from build123d import *

# Parameters (mm, degrees)
SKETCH1_R                          = 61.595
BOSS_EXTRUDE1_DEPTH                = 1.5875
F_1_4_0_25_DIAMETER_HOLE1_D        = 6.35
F_5_16_0_3125_DIAMETER_HOLE1_D     = 7.9375
F_5_16_0_3125_DIAMETER_HOLE1_DEPTH = 3.302


with BuildPart() as part:
    # Sketch1 → Boss-Extrude1 (new body, symmetric)
    with BuildSketch(Plane.XY):
        Circle(SKETCH1_R)
    extrude(amount=BOSS_EXTRUDE1_DEPTH, both=True)

    # 1/4 (0.25) Diameter Hole1 (through all)
    with Locations(Plane.XY.offset(1.5875)):
        with Locations((-47.625, 0), (47.625, 0)):
            Hole(F_1_4_0_25_DIAMETER_HOLE1_D / 2)

    # 5/16 (0.3125) Diameter Hole1
    with Locations(Plane.XY.offset(1.5875)):
        with Locations((0, 0)):
            Hole(F_5_16_0_3125_DIAMETER_HOLE1_D / 2, depth=F_5_16_0_3125_DIAMETER_HOLE1_DEPTH)


solid = part.part
Verification items for the finished model (mm, model axes). Round coordinates to 2 decimals unless told otherwise and drop trailing zeros. Order: outer loops, then holes, each group sorted by start corner. A loop starts at its lowest first (then second) coordinate and runs counter-clockwise, first axis right, second up.
1. Section check A-A on x = 0. Record the cut outline in (y, z) (1 decimal).
Final values:
outline: (-61.6, -1.6) - (-4, -1.6) - (-4, 1.6) - (-61.6, 1.6) - close; (4, -1.6) - (61.6, -1.6) - (61.6, 1.6) - (4, 1.6) - close
2. Section check D-D on y = 32. Record the cut outline in (x, z).
Final values:
outline: (-52.63, -1.59) - (52.63, -1.59) - (52.63, 1.59) - (-52.63, 1.59) - close
3. Release check for a two-part mould opening along Y. For faces 1 (the flat face through (-1, -13, 1.588)), 2 (the cylindrical face through (44.597, 0.954, -0.022)), 3 (the cylindrical face through (-13.35, -60.13, 0.02)) record: +Y half, -Y half, draft (parallel to the pull), parting line (faces both ways), or undercut.
Final values:
face 1: draft
face 2: undercut
face 3: parting line
4. Thickness scan on L1, parallel to Y at x = -3, z = 0.4; L2, parallel to X at y = -38.5, z = 0.3; L3, parallel to Y at x = -26, z = -0.7. Record the ranges inside material, lowest first.
Final values:
L1: y = -61.52 to -2.6, 2.6 to 61.52
L2: x = -48.08 to 48.08
L3: y = -55.84 to 55.84
5. Section check B-B on y = 0. State how many separate pieces and enclosed holes the cut face has, then the cut area to 3 significant figures.
Final values:
separate pieces: 4
enclosed holes: 0
area: 326 mm2
6. Go/stop test with flat-tipped pins: P1, Ø5, axis at x = -47.625, y = 0, coming from the -Z side; P2, Ø1, axis at x = 33.5, z = 0, coming from the -Y side. Record where each tip stops, or that it passes through.
Final values:
P1: passes through
P2: stops at y = -52.01
